from build123d import *

# Parameters (mm, degrees)
SKETCH4_W                      = 5
SKETCH4_H                      = 3.5
BOSS_EXTRUDE4_DEPTH            = 25
SKETCH8_W                      = 5
SKETCH8_H                      = 6
BOSS_EXTRUDE6_DEPTH            = 6
BOSS_EXTRUDE8_DEPTH            = 7
BOSS_EXTRUDE8_DEPTH_BACK       = 7
SKETCH10_W                     = 7
SKETCH10_H                     = 4
CUT_EXTRUDE1_REACH             = 19.869
SKETCH11_R                     = 0.86
CUT_EXTRUDE3_REACH             = 29.094
SKETCH5_R                      = 1.75
CUT_EXTRUDE3_DIRECTION_2_REACH = 29.094
CUT_EXTRUDE2_REACH             = 29.094
SKETCH9_R                      = 1.75
CUT_EXTRUDE2_DIRECTION_2_REACH = 29.094
CUT_EXTRUDE4_REACH             = 29.094
CUT_EXTRUDE4_END_RADIUS        = 1.75
SKETCH13_R                     = 1.1
CUT_EXTRUDE5_REACH             = 29.094
CUT_EXTRUDE5_END_RADIUS        = 1.75
SKETCH14_R                     = 1.1
RIB5_REACH                     = 29.844
SKETCH19_WALL_W                = 65.188868008
SKETCH19_WALL_H                = 5
RIB8_REACH                     = 29.645
SKETCH20_WALL_W                = 62.444026
SKETCH20_WALL_H                = 3.5
RIB9_REACH                     = 29.645
SKETCH21_WALL_W                = 62.444026
SKETCH21_WALL_H                = 3.5
FILLET2_R                      = 1


with BuildPart() as part:
    # Sketch4 → Boss-Extrude4 (new body)
    with BuildSketch(Plane(origin=(0, 0, 0), x_dir=(1, 0, 0), z_dir=(0, 1, 0))):
        Rectangle(SKETCH4_W, SKETCH4_H)
    extrude(amount=BOSS_EXTRUDE4_DEPTH)

    # Sketch8 → Boss-Extrude6 (add)
    with BuildSketch(Plane.XY.offset(1.75)):
        with Locations((0, 22)):
            Rectangle(SKETCH8_W, SKETCH8_H)
    extrude(amount=BOSS_EXTRUDE6_DEPTH)

    # Sketch10 → Boss-Extrude8 (add, two sides: drawn at the far end of the back side and taken through both)
    with BuildSketch(Plane(origin=(0, 0, 0), x_dir=(0, 0, -1), z_dir=(1, 0, 0)).offset(-BOSS_EXTRUDE8_DEPTH_BACK)):
        with Locations((-1.75, 12.5)):
            Rectangle(SKETCH10_W, SKETCH10_H)
    extrude(amount=BOSS_EXTRUDE8_DEPTH + BOSS_EXTRUDE8_DEPTH_BACK)

    # Sketch11 → Cut-Extrude1 (cut, up to next)
    with BuildSketch(Plane.XZ.offset(-10.5), mode=Mode.PRIVATE) as cut_extrude1_sk1:
        with Locations(Location((-5.3, 2.3, 0), (0, 0, 270))):
            Circle(SKETCH11_R)
    cut_extrude1_tool1 = extrude(cut_extrude1_sk1.sketch, amount=-CUT_EXTRUDE1_REACH, mode=Mode.PRIVATE) & part.part
    # Sketch11 → Cut-Extrude1 (cut, up to next)
    with BuildSketch(Plane.XZ.offset(-10.5), mode=Mode.PRIVATE) as cut_extrude1_sk2:
        with Locations(Location((4.72, 0.68, 0), (0, 0, 270))):
            Circle(SKETCH11_R)
    cut_extrude1_tool2 = extrude(cut_extrude1_sk2.sketch, amount=-CUT_EXTRUDE1_REACH, mode=Mode.PRIVATE) & part.part
    add(cut_extrude1_tool1.solids().sort_by_distance((-5.3, 10.5, 2.3))[0], mode=Mode.SUBTRACT)
    add(cut_extrude1_tool2.solids().sort_by_distance((4.72, 10.5, 0.68))[0], mode=Mode.SUBTRACT)

    # Sketch5 → Cut-Extrude3 (cut, up to next)
    with BuildSketch(Plane.XY, mode=Mode.PRIVATE) as cut_extrude3_sk1:
        with Locations(Location((0, 3, 0), (0, 0, 180))):
            Circle(SKETCH5_R)
    cut_extrude3_tool1 = extrude(cut_extrude3_sk1.sketch, amount=-CUT_EXTRUDE3_REACH, mode=Mode.PRIVATE) & part.part
    add(cut_extrude3_tool1.solids().sort_by_distance((0, 3, 0))[0], mode=Mode.SUBTRACT)

    # Sketch5 → Cut-Extrude3 direction 2 (cut, up to next)
    with BuildSketch(Plane.XY, mode=Mode.PRIVATE) as cut_extrude3_direction_2_sk1:
        with Locations(Location((0, 3, 0), (0, 0, 180))):
            Circle(SKETCH5_R)
    cut_extrude3_direction_2_tool1 = extrude(cut_extrude3_direction_2_sk1.sketch, amount=CUT_EXTRUDE3_DIRECTION_2_REACH, mode=Mode.PRIVATE) & part.part
    add(cut_extrude3_direction_2_tool1.solids().sort_by_distance((0, 3, 0))[0], mode=Mode.SUBTRACT)

    # Sketch9 → Cut-Extrude2 (cut, up to next)
    with BuildSketch(Plane.ZY, mode=Mode.PRIVATE) as cut_extrude2_sk1:
        with Locations((5, 22)):
            Circle(SKETCH9_R)
    cut_extrude2_tool1 = extrude(cut_extrude2_sk1.sketch, amount=CUT_EXTRUDE2_REACH, mode=Mode.PRIVATE) & part.part
    add(cut_extrude2_tool1.solids().sort_by_distance((0, 22, 5))[0], mode=Mode.SUBTRACT)

    # Sketch9 → Cut-Extrude2 direction 2 (cut, up to next)
    with BuildSketch(Plane.ZY, mode=Mode.PRIVATE) as cut_extrude2_direction_2_sk1:
        with Locations((5, 22)):
            Circle(SKETCH9_R)
    cut_extrude2_direction_2_tool1 = extrude(cut_extrude2_direction_2_sk1.sketch, amount=-CUT_EXTRUDE2_DIRECTION_2_REACH, mode=Mode.PRIVATE) & part.part
    add(cut_extrude2_direction_2_tool1.solids().sort_by_distance((0, 22, 5))[0], mode=Mode.SUBTRACT)

    # Cut-Extrude4: up to this cylinder (the profile starts outside it)
    cut_extrude4_end = Plane(origin=(0, 22, 5), z_dir=(-1, 0, 0)) * Cylinder(CUT_EXTRUDE4_END_RADIUS, 62.688, mode=Mode.PRIVATE)
    # Sketch13 → Cut-Extrude4 (cut, up to the surface)
    with BuildSketch(Plane(origin=(0, 25, 0), x_dir=(1, 0, 0), z_dir=(0, 1, 0)), mode=Mode.PRIVATE) as cut_extrude4_sk1:
        with Locations(Location((0, -5, 0), (0, 0, 270))):
            Circle(SKETCH13_R)
    cut_extrude4_tool1 = extrude(cut_extrude4_sk1.sketch, amount=-CUT_EXTRUDE4_REACH, mode=Mode.PRIVATE) - cut_extrude4_end
    add(cut_extrude4_tool1.solids().sort_by_distance((0, 25, 5))[0], mode=Mode.SUBTRACT)

    # Cut-Extrude5: up to this cylinder (the profile starts outside it)
    cut_extrude5_end = Plane(origin=(0, 3, 0), z_dir=(0, 0, -1)) * Cylinder(CUT_EXTRUDE5_END_RADIUS, 62.688, mode=Mode.PRIVATE)
    # Sketch14 → Cut-Extrude5 (cut, up to the surface)
    with BuildSketch(Plane.XZ, mode=Mode.PRIVATE) as cut_extrude5_sk1:
        with Locations(Location((0, 0, 0), (0, 0, 270))):
            Circle(SKETCH14_R)
    cut_extrude5_tool1 = extrude(cut_extrude5_sk1.sketch, amount=-CUT_EXTRUDE5_REACH, mode=Mode.PRIVATE) - cut_extrude5_end
    add(cut_extrude5_tool1.solids().sort_by_distance((0, 0, 0))[0], mode=Mode.SUBTRACT)

    # Sketch19 wall → Rib5 (add, up to next)
    with BuildSketch(Plane(origin=(-2.5, 16.75, 4.75), x_dir=(0, 0.6, 0.8), z_dir=(0, 0.8, -0.6)), mode=Mode.PRIVATE) as rib5_sk1:
        with Locations((0, 2.5)):
            Rectangle(SKETCH19_WALL_W, SKETCH19_WALL_H)
    rib5_tool1 = extrude(rib5_sk1.sketch, amount=RIB5_REACH, mode=Mode.PRIVATE) - part.part
    add(rib5_tool1.solids().sort_by_distance((-2.5, 16.75, 4.75))[0])

    # Sketch20 wall → Rib8 (add, up to next)
    with BuildSketch(Plane(origin=(-3.125, 17, -1.75), x_dir=(-0.242535625036, -0.970142500145, 0), z_dir=(-0.970142500145, 0.242535625036, 0)), mode=Mode.PRIVATE) as rib8_sk1:
        with Locations((0, 1.75)):
            Rectangle(SKETCH20_WALL_W, SKETCH20_WALL_H)
    rib8_tool1 = extrude(rib8_sk1.sketch, amount=-RIB8_REACH, mode=Mode.PRIVATE) - part.part
    rib8 = rib8_tool1.solids().sort_by_distance((-3.125, 17, -1.75))[0]
    add(rib8)

    # Sketch21 wall → Rib9 (add, up to next)
    with BuildSketch(Plane(origin=(-3.125, 8, -1.75), x_dir=(0.242535625036, -0.970142500145, 0), z_dir=(-0.970142500145, -0.242535625036, 0)), mode=Mode.PRIVATE) as rib9_sk1:
        with Locations((0, 1.75)):
            Rectangle(SKETCH21_WALL_W, SKETCH21_WALL_H)
    rib9_tool1 = extrude(rib9_sk1.sketch, amount=-RIB9_REACH, mode=Mode.PRIVATE) - part.part
    rib9 = rib9_tool1.solids().sort_by_distance((-3.125, 8, -1.75))[0]
    add(rib9)

    # Mirror3: Rib8, Rib9 across plane
    add(rib8.mirror(Plane(origin=(0, 0, 0), x_dir=(0, 0, 1), z_dir=(1, 0, 0))))
    add(rib9.mirror(Plane(origin=(0, 0, 0), x_dir=(0, 0, 1), z_dir=(1, 0, 0))))

    # Fillet2
    # the kernel refuses this fillet: 1 mm, written as the material it adds along each edge
    with BuildSketch(Plane(origin=(-2.5, 19.5, 1.75), x_dir=(-0.2425356250360274, -0.9701425001454083, 0), z_dir=(0, 0, -1)), Plane(origin=(-2.5, 5.5, -1.75), x_dir=(-0.24253562503611567, 0.9701425001453862, 0), z_dir=(0, 0, 1)), Plane(origin=(2.5, 5.5, -1.75), x_dir=(0, -1, 0), z_dir=(0, 0, 1))) as fillet2_piece_1:
        with BuildLine():
            CenterArc((FILLET2_R * 0.123105625617, FILLET2_R), FILLET2_R, 255.963756532, 14.036243468)
            Line((-FILLET2_R * 0.119429999419, FILLET2_R * 0.0298574998546), (0, 0))
            Line((0, 0), (FILLET2_R * 0.123105625618, 0))
        make_face()
    fillet2_piece_1_solid = extrude(amount=3.5, mode=Mode.PRIVATE)
    with BuildSketch(Plane(origin=(2.5, 19.5, 1.75), x_dir=(0.24253562503603418, -0.9701425001454065, 0), z_dir=(0, 0, -1))) as fillet2_piece_2:
        with BuildLine():
            CenterArc((FILLET2_R * 0.123105625617, -FILLET2_R), FILLET2_R, 90, 14.036243468)
            Line((-FILLET2_R * 0.119429999419, -FILLET2_R * 0.0298574998546), (0, 0))
            Line((0, 0), (FILLET2_R * 0.123105625618, 0))
        make_face()
    fillet2_piece_2_solid = extrude(amount=3.5, mode=Mode.PRIVATE)
    add([fillet2_piece_1_solid, fillet2_piece_2_solid])
    # the kernel refuses this fillet: 1 mm, written as the material it takes off along each edge
    with BuildSketch(Plane(origin=(-2.5, 25, 10.25), x_dir=(0, -1, 0), z_dir=(0, 0, -1)), Plane(origin=(2.5, 25, -4.25), x_dir=(0, -1, 0), z_dir=(0, 0, 1))) as fillet2_2_piece_1:
        with BuildLine():
            CenterArc((FILLET2_R, -FILLET2_R), FILLET2_R, 90, 90)
            Line((0, -FILLET2_R), (0, 0))
            Line((0, 0), (FILLET2_R, 0))
        make_face()
    fillet2_2_piece_1_solid = extrude(amount=14.5, mode=Mode.PRIVATE)
    with BuildSketch(Plane(origin=(3.75, 19, 7.75), x_dir=(0, -0.5999999999999996, -0.8000000000000002), z_dir=(-1, 0, 0))) as fillet2_2_piece_2:
        with BuildLine():
            CenterArc((FILLET2_R * 0.5, -FILLET2_R), FILLET2_R, 90, 53.130102354)
            Line((-FILLET2_R * 0.3, -FILLET2_R * 0.4), (0, 0))
            Line((0, 0), (FILLET2_R * 0.5, 0))
        make_face()
    fillet2_2_piece_2_solid = extrude(amount=7.5, mode=Mode.PRIVATE)
    with BuildSketch(Plane(origin=(-5, 25, 7.75), x_dir=(0, 0, -1), z_dir=(1, 0, 0)), Plane(origin=(-5, 0, 1.75), x_dir=(0, 1, 0), z_dir=(1, 0, 0))) as fillet2_2_piece_3:
        with BuildLine():
            CenterArc((FILLET2_R, -FILLET2_R), FILLET2_R, 90, 90)
            Line((0, -FILLET2_R), (0, 0))
            Line((0, 0), (FILLET2_R, 0))
        make_face()
    fillet2_2_piece_3_solid = extrude(amount=10, mode=Mode.PRIVATE)
    with BuildSketch(Plane(origin=(-7, 14.5, -4.25), x_dir=(0, -1, 0), z_dir=(0, 0, 1)), Plane(origin=(7, 10.5, 7.75), x_dir=(-1, 0, 0), z_dir=(0, 0, -1))) as fillet2_2_piece_4:
        with BuildLine():
            CenterArc((FILLET2_R, FILLET2_R), FILLET2_R, 180, 90)
            Line((0, FILLET2_R), (0, 0))
            Line((0, 0), (FILLET2_R, 0))
        make_face()
    fillet2_2_piece_4_solid = extrude(amount=12, mode=Mode.PRIVATE)
    with BuildSketch(Plane(origin=(9.5, 10.5, 5.25), x_dir=(0, 0, -1), z_dir=(-1, 0, 0)), Plane(origin=(9.5, 14.5, 5.25), x_dir=(0, -1, 0), z_dir=(-1, 0, 0))) as fillet2_2_piece_5:
        with BuildLine():
            CenterArc((FILLET2_R, -FILLET2_R), FILLET2_R, 90, 90)
            Line((0, -FILLET2_R), (0, 0))
            Line((0, 0), (FILLET2_R, 0))
        make_face()
    fillet2_2_piece_5_solid = extrude(amount=19, mode=Mode.PRIVATE)
    with BuildSketch(Plane(origin=(-7, 10.5, 7.75), x_dir=(1, 0, 0), z_dir=(0, 0, -1)), Plane(origin=(7, 14.5, -4.25), x_dir=(0, -1, 0), z_dir=(0, 0, 1))) as fillet2_2_piece_6:
        with BuildLine():
            CenterArc((FILLET2_R, -FILLET2_R), FILLET2_R, 90, 90)
            Line((0, -FILLET2_R), (0, 0))
            Line((0, 0), (FILLET2_R, 0))
        make_face()
    fillet2_2_piece_6_solid = extrude(amount=12, mode=Mode.PRIVATE)
    with BuildSketch(Plane(origin=(-2.5, 0, -4.25), x_dir=(1, 0, 0), z_dir=(0, 0, 1)), Plane(origin=(2.5, 0, 4.25), x_dir=(-1, 0, 0), z_dir=(0, 0, -1))) as fillet2_2_piece_7:
        with BuildLine():
            CenterArc((FILLET2_R, FILLET2_R), FILLET2_R, 180, 90)
            Line((0, FILLET2_R), (0, 0))
            Line((0, 0), (FILLET2_R, 0))
        make_face()
    fillet2_2_piece_7_solid = extrude(amount=8.5, mode=Mode.PRIVATE)
    add([fillet2_2_piece_1_solid, fillet2_2_piece_2_solid, fillet2_2_piece_3_solid, fillet2_2_piece_4_solid, fillet2_2_piece_5_solid, fillet2_2_piece_6_solid, fillet2_2_piece_7_solid], mode=Mode.SUBTRACT)


solid = part.part
Verification items for the finished model (mm, model axes). A direction names the side the tool comes from. Round coordinates to 2 decimals unless told otherwise and drop trailing zeros. Loops run counter-clockwise (first coordinate to the right, second up) from the corner with the lowest first, then second, coordinate; pieces in that order, holes last. Notation, with made-up numbers: (0.25, -30.5) - (19.25, -30.5) arc R11 cw to (19.25, -22.5) - close; hole circle Ø9 at (82.5, -38.75). An arc over 180 degrees is marked (long way). Use one line per item in the form item = value.
1. Gauge pin test, flat ends, axial feed: pin 1 Ø3.5 at (x, y) = (-1, 6) entering from +Z; pin 2 Ø4 at (y, z) = (2, -0.5) entering from +X; pin 3 Ø2 at (x, z) = (-5.3, 2.3) entering from -Y. Record the tip position at first contact, or that the pin passes through.
A:
pin_1 = 1.75
pin_2 = 2.5
pin_3 = 10.5
2. Section check B-B on x = -5.3. Record the cut outline in (y, z), and give its area (3 significant figures).
A:
outline = (10.5, -1.75) - (14.5, -1.75) - (14.5, 1.44) - (10.5, 1.44) - close; (10.5, 3.16) - (14.5, 3.16) - (14.5, 4.25) arc R1 ccw to (13.5, 5.25) - (11.5, 5.25) arc R1 ccw to (10.5, 4.25) - close
area = 20.7 mm²
3. Section check A-A on y = 22. Record the cut outline in (x, z), and give its area (3 significant figures).
A:
outline = (-2.5, -1.75) - (2.5, -1.75) - (2.5, 3.25) - (-2.5, 3.25) - close; (-2.5, 6.75) - (2.5, 6.75) - (2.5, 7.75) - (-2.5, 7.75) - close
area = 30.0 mm²
4. Scan lines: probe 1 along Z at (x, y) = (0, 1.05); probe 2 along Y at (x, z) = (1.25, 4.5); probe 3 along X at (y, z) = (3, -0.8). Record each from-to range of solid material in increasing order.
A:
probe_1 = -1.75 to -1.1, 1.1 to 1.75
probe_2 = 10.53 to 14.47, 16.56 to 20.32, 23.68 to 25
probe_3 = -2.5 to -1.75, 1.75 to 2.5
5. Section check C-C on x = 0.5. Record the cut outline in (y, z), and give its area (3 significant figures).
A:
outline = (0, -1.75) - (1.32, -1.75) - (1.32, -0.98) - (0, -0.98) - close; (0.03, 0.98) - (1.32, 0.98) - (1.32, 1.75) - (1, 1.75) arc R1 ccw to start; (4.68, -1.75) - (25, -1.75) - (25, 4.02) - (23.45, 4.02) arc R1.75 cw (long way) to (23.45, 5.98) - (25, 5.98) - (25, 6.75) arc R1 ccw to (24, 7.75) - (19.5, 7.75) arc R1 ccw to (18.7, 7.35) - (14.5, 1.75) - (14.5, 4.25) arc R1 ccw to (13.5, 5.25) - (11.5, 5.25) arc R1 ccw to (10.5, 4.25) - (10.5, 1.75) - (4.68, 1.75) - close
area = 124 mm²
6. Section check D-D on z = 2.3. Record the cut outline in (x, y).
A:
outline = (-7, 11.5) arc R1 ccw to (-6.16, 10.51) - (-6.16, 14.49) arc R1 ccw to (-7, 13.5) - close; (-4.44, 10.5) - (6, 10.5) arc R1 ccw to (7, 11.5) - (7, 13.5) arc R1 ccw to (6, 14.5) - (-4.44, 14.5) - close; (-2.5, 14.91) - (2.5, 14.91) - (2.5, 24) arc R1 ccw to (1.5, 25) - (-1.5, 25) arc R1 ccw to (-2.5, 24) - close
7. Draft check along Y on faces 1 (the flat face through (0, 25, 2)), 2 (the flat face through (0, 12, -1.75)), 3 (the cylindrical face through (0.38, 4.71, 0.02)), 4 (the flat face through (-3.148, 8.094, 0.024)). Enter one of: pulls with the +Y half, pulls with the -Y half, needs draft (parallel to the pull), parting line crosses it, or undercut.
A:
face_1 = pulls with the +Y half
face_2 = needs draft
face_3 = undercut
face_4 = pulls with the -Y half
8. Access from +Z, -Z, +X, -X, +Y, -Y to the whole of each face (thin tool, end or side, straight path). Record for faces 5 (the flat face through (-2.5, 3, 0)), 6 (the cylindrical face through (0.098, 14.199, 4.965)), 7 (the flat face through (2.5, 3, 0)), 8 (the flat face through (2.5, 20, 3)), 9 (the flat face through (0, 12, 5.25)).
A:
face_5 = +Z, -Z, -X, -Y
face_6 = +Z, +X, -X
face_7 = +Z, -Z, +X, -Y
face_8 = +Z, +X, +Y
face_9 = +Z, +X, -X, -Y
